The listing builds one solid part. Answer for the finished solid, in the listing's coordinates (mm). A direction names the side the tool comes from. Round coordinates to 2 decimals unless told otherwise and drop trailing zeros. Order: outer loops, then holes, each group sorted by start corner. A loop starts at its lowest first (then second) coordinate and runs counter-clockwise, first axis right, second up. Notation, with made-up numbers: (33.25, 27) - (46.25, 27) arc R7 ccw to (46.25, 36) - close; hole circle Ø5 at (-7, -18). An arc over 180 degrees is marked (long way). Write item = value, one per line.
from build123d import *

# Parameters (mm, degrees)
SKETCH1_R               = 90
BOSS_EXTRUDE1_DEPTH     = 100
CUT_EXTRUDE1_DEPTH      = 200
CUT_EXTRUDE1_DEPTH_BACK = 200
SKETCH2_W               = 61
SKETCH2_H               = 70
CUT_EXTRUDE2_DEPTH      = 200
CUT_EXTRUDE2_DEPTH_BACK = 200
SKETCH3_R               = 10


with BuildPart() as part:
    # Sketch1 → Boss-Extrude1 (new body)
    with BuildSketch(Plane.XY):
        Circle(SKETCH1_R)
    extrude(amount=BOSS_EXTRUDE1_DEPTH)

    # Sketch2 → Cut-Extrude1 (cut, two sides: drawn at the far end of the back side and taken through both)
    with BuildSketch(Plane(origin=(0, 0, 0), x_dir=(1, 0, 0), z_dir=(0, 1, 0)).offset(-CUT_EXTRUDE1_DEPTH_BACK)):
        with Locations((0, -65)):
            Rectangle(SKETCH2_W, SKETCH2_H)
    extrude(amount=CUT_EXTRUDE1_DEPTH + CUT_EXTRUDE1_DEPTH_BACK, mode=Mode.SUBTRACT)

    # Sketch3 → Cut-Extrude2 (cut, two sides: drawn at the far end of the back side and taken through both)
    with BuildSketch(Plane(origin=(0, 0, 0), x_dir=(0, 0, -1), z_dir=(1, 0, 0)).offset(-CUT_EXTRUDE2_DEPTH_BACK)):
        with Locations((0, 70)):
            Circle(SKETCH3_R)
    extrude(amount=CUT_EXTRUDE2_DEPTH + CUT_EXTRUDE2_DEPTH_BACK, mode=Mode.SUBTRACT)


solid = part.part
Q1. Section D-D on z = 17 is taken. Determine the outline of the cut face in (x, y), then the cut area to 3 significant figures.
Model answer:
outline = circle Ø180 at (0, 0)
area = 25,400 mm^2
Q2. Section C-C on x = 17.5 is taken. Determine the outline of the cut face in (y, z), then the cut area to 3 significant figures.
Model answer:
outline = (-88.28, 0) - (60, 0) arc R10 cw to (80, 0) - (88.28, 0) - (88.28, 30) - (-88.28, 30) - close
area = 5,140 mm^2
Q3. Flat-ended cylindrical pins translate along their axes: P1, Ø8, axis at y = -62.5, z = 55, coming from the +X side; P2, Ø1.5, axis at x = -20.5, z = 18.5, coming from the -Y side; P3, Ø4, axis at y = -57.5, z = 51, coming from the -X side. Find the tip coordinate at first contact, or state that the pin passes through.
Model answer:
P1 = 68.39
P2 = -87.81
P3 = -70.85
Q4. Section A-A on z = 77.5 is taken. Determine the outline of the cut face in (x, y), then the cut area to 3 significant figures.
Model answer:
outline = (-30.5, -84.67) - (-30.5, 84.67) arc R90 ccw to start; (30.5, -84.67) arc R90 ccw to (30.5, 84.67) - close
area = 14,700 mm^2
Q5. Section B-B on y = 0 is taken. Determine the outline of the cut face in (x, z), then the cut area to 3 significant figures.
Model answer:
outline = (-90, 0) - (90, 0) - (90, 100) - (30.5, 100) - (30.5, 30) - (-30.5, 30) - (-30.5, 100) - (-90, 100) - close
area = 13,700 mm^2
Q6. Find the intervals of material crossed by line 1 (Z direction, x = 21, y = 32); line 2 (X direction, y = -49, z = 41.5); line 3 (X direction, y = -1, z = 89.5), in increasing order. Write a range as from..to.
Model answer:
line_1 = 0..30
line_2 = -75.49..-30.5, 30.5..75.49
line_3 = -89.99..-30.5, 30.5..89.99
Q7. For faces 4 (the face through (-1, -14, 0)), 5 (the face through (-30.5, -1, 65)), determine the directions among +Z, -Z, +X, -X, +Y, -Y from which every point of the face is accessible in a straight line to the end or side of a thin tool.
Model answer:
face_4 = -Z, +X, -X, +Y, -Y
face_5 = +Z, +Y, -Y
Q8. Determine the mould class of faces 1 (the face through (-0.94, 66.79, 9.47)), 2 (the face through (0, -1, 30)), 3 (the face through (83.137, -34.471, 49.3)) for opening direction Y: released by +Y, released by -Y, zero draft, split by the parting line, or undercut.
Model answer:
face_1 = undercut
face_2 = zero draft
face_3 = split by the parting line
